```python
from build123d import *

# Parameters (mm, degrees)
SKETCH_1_W          = 47
SKETCH_1_H          = 38
SKETCH_1_R          = 1.5
SKETCH_1_R_2        = 2.1
EXTRUDE_1_DEPTH     = 8
SKETCH_2_R          = 3.75
SKETCH_2_W          = 30
SKETCH_2_H          = 10
CUT_EXTRUDE_1_DEPTH = 4.5
SKETCH_3_W          = 47
SKETCH_3_H          = 10
EXTRUDE_2_DEPTH     = 5
CUT_EXTRUDE_2_DEPTH = 6
SKETCH_5_R          = 1.5
CUT_EXTRUDE_3_DEPTH = 6
SKETCH_6_R          = 1.5
CUT_EXTRUDE_4_DEPTH = 6
CUT_EXTRUDE_START   = -6
SKETCH_7_R          = 1.5
CUT_EXTRUDE_5_DEPTH = 6
SKETCH_8_R          = 1.5
CUT_EXTRUDE_6_DEPTH = 62.822326064


with BuildPart() as part:
    # Sketch 1 → Extrude 1 (new body)
    with BuildSketch(Plane.XY):
        with Locations((23.5, 19)):
            Rectangle(SKETCH_1_W, SKETCH_1_H)
        with Locations((16.25, 34)):
            Circle(SKETCH_1_R, mode=Mode.SUBTRACT)
        with Locations(Location((30.75, 34, 0), (0, 0, 180))):
            Circle(SKETCH_1_R, mode=Mode.SUBTRACT)
        with Locations((32.75, 14.75)):
            Circle(SKETCH_1_R_2, mode=Mode.SUBTRACT)
        with Locations(Location((14.25, 14.75, 0), (0, 0, 180))):
            Circle(SKETCH_1_R_2, mode=Mode.SUBTRACT)
        with Locations((11.5, 34)):
            Circle(SKETCH_1_R, mode=Mode.SUBTRACT)
        with Locations(Location((35.5, 34, 0), (0, 0, 180))):
            Circle(SKETCH_1_R, mode=Mode.SUBTRACT)
    extrude(amount=EXTRUDE_1_DEPTH)

    # Sketch 2 → Cut-Extrude 1 (cut)
    with BuildSketch(Plane(origin=(0, 0, 0), x_dir=(-1, 0, 0), z_dir=(0, 0, -1))):
        with Locations((-32.75, 14.75)):
            Circle(SKETCH_2_R)
        with Locations((-14.25, 14.75)):
            Circle(SKETCH_2_R)
        with Locations((-23.5, 5)):
            Rectangle(SKETCH_2_W, SKETCH_2_H)
    extrude(amount=-CUT_EXTRUDE_1_DEPTH, mode=Mode.SUBTRACT)

    # Sketch 3 → Extrude 2 (add)
    with BuildSketch(Plane.XY.offset(8)):
        with Locations((23.5, 5)):
            Rectangle(SKETCH_3_W, SKETCH_3_H)
    extrude(amount=EXTRUDE_2_DEPTH)

    # Sketch 4 → Cut-Extrude 2 (cut)
    with BuildSketch(Plane.XZ):
        Polygon((0.499880505, 7), (0, 8), (0, 6), (47, 6), (47, 7.999217306), (44.9861953, 7.999292351), (44, 8.985487652), (44, 10.499664551), (42.641699926, 13), (39.504118259, 13), (38, 10.499670662), (38, 9.249505993), (36.882697476, 7.999594333), (25.996893132, 8), (25.496893132, 8), (24.997012627, 7), (24.497012627, 7), (23.997132122, 8), (23.497132122, 8), (22.997251617, 7), (22.497251617, 7), (21.997371111, 8), (21.497371111, 8), (20.997490606, 7), (20.497490606, 7), (19.997610101, 8), (19.497610101, 8), (18.997729596, 7), (18.497729596, 7), (17.997849091, 8), (17.497849091, 8), (16.997968586, 7), (16.497968586, 7), (15.998088081, 8), (15.498088081, 8), (14.998207576, 7), (14.498207576, 7), (13.998327071, 8), (13.498327071, 8), (12.998446566, 7), (12.498446566, 7), (11.998566061, 8), (11.498566061, 8), (10.998685556, 7), (10.498685556, 7), (9.998805051, 8), (9.498805051, 8), (8.998924546, 7), (8.498924546, 7), (7.999044041, 8), (7.499044041, 8), (6.999163535, 7), (6.499163535, 7), (5.99928303, 8), (5.49928303, 8), (4.999402525, 7), (4.499402525, 7), (3.99952202, 8), (3.49952202, 8), (2.999641515, 7), (2.499641515, 7), (1.99976101, 8), (1.49976101, 8), (0.999880505, 7), align=None)
    extrude(amount=-CUT_EXTRUDE_2_DEPTH, mode=Mode.SUBTRACT)

    # Sketch 5 → Cut-Extrude 3 (cut)
    with BuildSketch(Plane(origin=(0, 0, 0), x_dir=(-1, 0, 0), z_dir=(0, 0, -1))):
        with Locations((-41.288047011, 3.201203266)):
            Circle(SKETCH_5_R)
    extrude(amount=-CUT_EXTRUDE_3_DEPTH, mode=Mode.SUBTRACT)

    # Sketch 6 → Cut-Extrude 4 (cut)
    with BuildSketch(Plane(origin=(47, 0, 0), x_dir=(0, 0, -1), z_dir=(1, 0, 0))):
        with Locations((-4, 12)):
            Circle(SKETCH_6_R)
        with Locations((-4, 20)):
            Circle(SKETCH_6_R)
        with Locations((-4, 28)):
            Circle(SKETCH_6_R)
    extrude(amount=-CUT_EXTRUDE_4_DEPTH, mode=Mode.SUBTRACT)

    # Sketch 7 → Cut-Extrude 5 (cut)
    with BuildSketch(Plane.ZY.offset(CUT_EXTRUDE_START)):
        with Locations(Location((4, 12, 0), (0, 0, 180))):
            Circle(SKETCH_7_R)
        with Locations(Location((4, 20, 0), (0, 0, 180))):
            Circle(SKETCH_7_R)
        with Locations(Location((4, 28, 0), (0, 0, 180))):
            Circle(SKETCH_7_R)
    extrude(amount=CUT_EXTRUDE_5_DEPTH, mode=Mode.SUBTRACT)

    # Sketch 8 → Cut-Extrude 6 (cut, through all)
    with BuildSketch(Plane(origin=(0, 0, 0), x_dir=(-1, 0, 0), z_dir=(0, 0, -1))):
        with Locations((-40.861215873, 16.298578495)):
            Circle(SKETCH_8_R)
        with Locations((-40.861215873, 24.11472755)):
            Circle(SKETCH_8_R)
        with Locations((-6.138784127, 16.298578495)):
            Circle(SKETCH_8_R)
        with Locations((-6.138784127, 24.11472755)):
            Circle(SKETCH_8_R)
    extrude(amount=-CUT_EXTRUDE_6_DEPTH, mode=Mode.SUBTRACT)


solid = part.part
```
Model file for the job. Use its own axes, mm. A direction names the side the tool comes from. Give positions to 0.01 mm unless a question says otherwise; leave off trailing zeros. Loops run counter-clockwise (first coordinate to the right, second up) from the corner with the lowest first, then second, coordinate; pieces in that order, holes last. Notation, with made-up numbers: (48, 57) -> (61, 57) arc R28 cw to (61, 86) -> close; hole circle Ø8 at (-2.5, -37.75). An arc over 180 degrees is marked (long way). Use CSV: the item, a comma, the result in double quotes. Start each with the question number.
1) Flat gauge pins, fed straight in: pin 1 Ø3.5 at (y, z) = (4, 1.5) entering from -X; pin 2 Ø1.8 at (y, z) = (28, 4) entering from -X; pin 3 Ø0.6 at (x, y) = (12, 3) entering from -Z; pin 4 Ø2.5 at (x, y) = (40.86, 16.3) entering from -Z (1 decimal). Where does each tip first touch, or does it go through?
2) Slice it at B-B on x = 35.5. Give the cut face in (y, z), plus the area to 3 significant figures.
3) Slice it at C-C on z = 1. Give the number of separate pieces and of enclosed holes in the cut face, plus the area to 3 significant figures.
4) Wall check: line 1 (Y direction, x = 43.3, z = 4); line 2 (Z direction, x = 35.5, y = 3); line 3 (Y direction, x = 16, z = 5.25). Give the ranges that are in metal, low to high.
5) Slice it at D-D on y = 8. Give the cut face in (x, z).
6) Slice it at A-A on y = 34. Give the cut face in (x, z), plus the area to 3 significant figures.
7) Mould opens along Y. For faces 1 (the flat face through (4.253, 2.958, 7.493)), 2 (the flat face through (23, 0, 5)), 3 (the flat face through (41, 28, 4)) say: released by +Y, released by -Y, zero draft, split by the parting line, or undercut.
8) Tool access for faces 4 (the flat face through (23, 10, 10)), 5 (the flat face through (41, 20, 4)), 6 (the flat face through (23.25, 2.96, 7.51)): list every direction of +Z, -Z, +X, -X, +Y, -Y with a clear straight run to the whole face (end or side of a thin tool).
Computed values:
1,pin 1,"stops at x = 0"
1,pin 2,"stops at x = 6"
1,pin 3,"stops at z = 4.5"
1,pin 4,"passes through"
2,outline,"(0, 4.5) -> (10, 4.5) -> (10, 0) -> (12.2, 0) -> (12.2, 4.5) -> (17.3, 4.5) -> (17.3, 0) -> (32.5, 0) -> (32.5, 8) -> (10, 8) -> (10, 13) -> (0, 13) -> (0, 8) -> (6, 8) -> (6, 6) -> (0, 6) -> close; (35.5, 0) -> (38, 0) -> (38, 8) -> (35.5, 8) -> close"
2,area,"250 mm^2"
3,separate pieces,"1"
3,enclosed holes,"11"
3,area,"1,330 mm^2"
4,line 1,"y = 0 to 10.5, 13.5 to 18.5, 21.5 to 26.5, 29.5 to 38"
4,line 2,"z = 4.5 to 6, 8 to 13"
4,line 3,"y = 0 to 13.59, 15.91 to 32.52, 35.48 to 38"
5,outline,"(0, 0) -> (8.5, 0) -> (8.5, 4.5) -> (38.5, 4.5) -> (38.5, 0) -> (47, 0) -> (47, 13) -> (0, 13) -> close"
6,outline,"(0, 0) -> (10, 0) -> (10, 8) -> (0, 8) -> close; (13, 0) -> (14.75, 0) -> (14.75, 8) -> (13, 8) -> close; (17.75, 0) -> (29.25, 0) -> (29.25, 8) -> (17.75, 8) -> close; (32.25, 0) -> (34, 0) -> (34, 8) -> (32.25, 8) -> close; (37, 0) -> (47, 0) -> (47, 8) -> (37, 8) -> close"
6,area,"280 mm^2"
7,face 1,"zero draft"
7,face 2,"released by -Y"
7,face 3,"undercut"
8,face 4,"+Z, +X, -X, +Y"
8,face 5,"+X"
8,face 6,"-Y"
